```python
from build123d import *

# Parameters (mm, degrees)
BOSS_EXTRUDE1_DEPTH      = 16.51
SKETCH2_R                = 25.4
BOSS_EXTRUDE2_DEPTH      = 19.05
BOSS_EXTRUDE3_DEPTH      = 34.925
BOSS_EXTRUDE3_DEPTH_BACK = 34.925
SKETCH3_R                = 6.35
SKETCH3_2_R              = 6.35
CUT_EXTRUDE1_DEPTH       = 22.225


with BuildPart() as part:
    # Sketch1 → Boss-Extrude1 (new body)
    with BuildSketch(Plane(origin=(0, 0, 0), x_dir=(0, 0, -1), z_dir=(1, 0, 0))):
        with BuildLine():
            Line((-38.1, 0), (-38.1, 50.8))
            Line((-38.1, 50.8), (-12.7, 50.8))
            Line((-12.7, 50.8), (-12.7, 76.2))
            Line((-12.7, 76.2), (12.7, 76.2))
            Line((12.7, 76.2), (12.7, 50.8))
            Line((12.7, 50.8), (38.1, 50.8))
            Line((38.1, 50.8), (38.1, 0))
            ThreePointArc((38.1, 0), (0, -38.1), (-38.1, 0))
        make_face()
        Polygon((0, 25.4), (-21.997045256, 12.7), (-21.997045256, -12.7), (0, -25.4), (21.997045256, -12.7), (21.997045256, 12.7), align=None, mode=Mode.SUBTRACT)
    extrude(amount=BOSS_EXTRUDE1_DEPTH)

    # Sketch2 → Boss-Extrude2 (add)
    with BuildSketch(Plane(origin=(-32.995567884, 19.05, 0), x_dir=(0, 0, 1), z_dir=(0.8660254037844416, -0.49999999999999495, 0))):
        with BuildLine():
            Line((-12.7, -65.991135768), (12.7, -65.991135768))
            Line((12.7, -65.991135768), (12.7, -84.257067086))
            ThreePointArc((12.7, -84.257067086), (28.838369623, -97.090778855), (34.925, -116.791135768))
            Line((34.925, -116.791135768), (34.925, -173.941135768))
            Line((34.925, -173.941135768), (-34.925, -173.941135768))
            Line((-34.925, -173.941135768), (-34.925, -116.791135768))
            ThreePointArc((-34.925, -116.791135768), (-28.838369623, -97.090778855), (-12.7, -84.257067086))
            Line((-12.7, -84.257067086), (-12.7, -65.991135768))
        make_face()
        with Locations(Location((0, -116.791135768, 0), (0, 0, 270))):
            Circle(SKETCH2_R, mode=Mode.SUBTRACT)
    extrude(amount=BOSS_EXTRUDE2_DEPTH)

    # Sketch3 → Boss-Extrude3 (add, two sides: drawn at the far end of the back side and taken through both)
    with BuildSketch(Plane.XY.offset(-BOSS_EXTRUDE3_DEPTH_BACK)):
        with BuildLine():
            Line((53.975, 169.687442339), (31.977954744, 182.387442339))
            ThreePointArc((31.977954744, 182.387442339), (14.629432116, 177.73891971), (19.277954744, 160.390397082))
            Line((19.277954744, 160.390397082), (41.275, 147.690397082))
            Line((41.275, 147.690397082), (53.975, 169.687442339))
        make_face()
        with Locations((25.627954744, 171.38891971)):
            Circle(SKETCH3_R, mode=Mode.SUBTRACT)
    extrude(amount=BOSS_EXTRUDE3_DEPTH + BOSS_EXTRUDE3_DEPTH_BACK)

    # Sketch3_2 → Cut-Extrude1 (cut, symmetric)
    with BuildSketch(Plane.XY):
        with BuildLine():
            Line((53.975, 169.687442339), (31.977954744, 182.387442339))
            ThreePointArc((31.977954744, 182.387442339), (14.629432116, 177.73891971), (19.277954744, 160.390397082))
            Line((19.277954744, 160.390397082), (41.275, 147.690397082))
            Line((41.275, 147.690397082), (53.975, 169.687442339))
        make_face()
        with Locations((25.627954744, 171.38891971)):
            Circle(SKETCH3_2_R, mode=Mode.SUBTRACT)
    extrude(amount=CUT_EXTRUDE1_DEPTH, both=True, mode=Mode.SUBTRACT)


solid = part.part
```
Design review of the part built by this model. Coordinates are the model's own, in mm. A direction names the side the tool comes from. Round coordinates to 2 decimals unless told otherwise and drop trailing zeros. Write item = value, one per line. Start each with the question number.
1) Mouldability with a two-part tool opening along Z and no side actions: class faces 4 (the face through (33, 166, 22.225)), 5 (the face through (30.12, 154.13, 28.49)), 6 (the face through (8, 25, 38.1)) as +Z half, -Z half, draft (parallel to the pull), parting line (faces both ways), or undercut.
2) Tool access review of faces 1 (the face through (8, 70, -12.7)), 2 (the face through (8, 0, 21.997)), 3 (the face through (10, 71, 12.7)): name each direction out of +Z, -Z, +X, -X, +Y, -Y from which nothing blocks a thin tool from reaching the whole face with its end or side.
3) Clearance check with flat-ended pins moving along their axes: pin 1 (18 mm diameter, centred on x = 33, y = 159.5, fed in from +Z) (3 decimals); pin 2 (10 mm diameter, centred on y = 81.5, z = 4, fed in from -X); pin 3 (1 mm diameter, centred on y = 112, z = -28, fed in from -X); pin 4 (10 mm diameter, centred on x = 25.63, y = 171.39, fed in from +Z). State where each tip first meets the part, or that it passes through.
4) Take a section at A-A, the plane x = 29.5. Count the separate pieces of the cut face and the enclosed holes in it, plus the area to 3 significant figures.
5) Wall thickness on probe 1 along Z at (x, y) = (14.5, 169.5) (3 decimals); probe 2 along Y at (x, z) = (27.5, -31.5); probe 3 along Z at (x, y) = (22.5, 113): over which ranges is each line inside the solid? List them lowest first. Write a range as from..to.
Results list:
q1.face_4 = undercut
q1.face_5 = draft
q1.face_6 = +Z half
q2.face_1 = -Z, -X
q2.face_2 = +X, -X
q2.face_3 = +Z, -X
q3.pin_1 = 34.925
q3.pin_2 = 0.17
q3.pin_3 = 20.38
q3.pin_4 = through
q4.separate_pieces = 6
q4.enclosed_holes = 0
q4.area = 1,320 mm²
q5.probe_1 = -34.925..-22.225, 22.225..34.925
q5.probe_2 = 101.56..123.83, 155.64..165.32, 177.46..183.95
q5.probe_3 = -34.07..-24.21, 24.21..34.07
